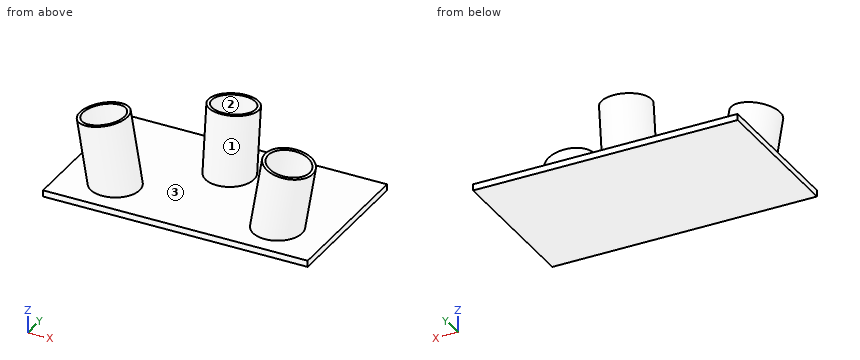
from build123d import *

# Parameters (mm, degrees)
F2_R      = 9.70750027
F2_R_2    = 8.43750027
F3_DEPTH  = 33.02
F4_DEPTH  = 50.8
F6_DEPTH  = 127
F8_R      = 9.70750027
F8_R_2    = 8.43750027
F9_DEPTH  = 33.02
F10_W     = 144.2738771439
F10_H     = 43.9907349646
F11_DEPTH = 381
F14_R     = 9.70750027
F14_R_2   = 8.43750027
F15_DEPTH = 25.4
F16_DEPTH = 50.8
F17_W     = 94.1894035786
F17_H     = 29.3832402676
F18_DEPTH = 127
F19_W     = 106.1688474409
F19_H     = 60.55200234
F20_DEPTH = 2.54


with BuildPart() as f3:
    # F2 (on line) → F3 (new body)
    with BuildSketch(Plane(origin=(0, 0, 0), x_dir=(0.9860251287, 0, 0.1665966554), z_dir=(0.1665966554, 0, -0.9860251287))):
        with Locations((-32.11030027, 38.1445123341)):
            Circle(F2_R)
        with Locations((-32.11030027, 38.1445123341)):
            Circle(F2_R_2, mode=Mode.SUBTRACT)
    extrude(amount=-F3_DEPTH)

    # F4 (add): a face of the model
    f4_faces = [f3.faces().sort_by_distance(p)[0] for p in [
        (-46.4636912241, -38.1445123341, 25.6375864152),
    ]]
    extrude(f4_faces, amount=-F4_DEPTH)

    # F5 (on Front) → F6 (cut, symmetric)
    with BuildSketch(Plane.XZ):
        Polygon((43.3516763151, 0), (0, 0), (-49.4034710573, 0), (-49.4034710573, -35.2993682027), (43.3516763151, -35.2993682027), align=None)
    extrude(amount=F6_DEPTH, both=True, mode=Mode.SUBTRACT)



with BuildPart() as f9:
    # F8 (on line) → F9 (new body)
    with BuildSketch(Plane(origin=(0, 0, 0), x_dir=(0.9860251287, 0, -0.1665966554), z_dir=(-0.1665966554, 0, -0.9860251287))):
        with Locations((32.11030027, 38.14450207)):
            Circle(F8_R)
        with Locations((32.11030027, 38.14450207)):
            Circle(F8_R_2, mode=Mode.SUBTRACT)
    extrude(amount=-F9_DEPTH)

    # F10 (on Front) → F11 (cut, symmetric)
    with BuildSketch(Plane.XZ):
        with Locations((2.6571601629, -21.9953674823)):
            Rectangle(F10_W, F10_H)
    extrude(amount=F11_DEPTH, both=True, mode=Mode.SUBTRACT)


with BuildPart() as f15:
    # F14 (on face) → F15 (new body)
    with BuildSketch(Plane(origin=(0, 0, 0), x_dir=(1, 0, 0), z_dir=(0, 0.1114689322, 0.9937679192))):
        with Locations((0, -12.55230027)):
            Circle(F14_R)
        with Locations((0, -12.55230027)):
            Circle(F14_R_2, mode=Mode.SUBTRACT)
    extrude(amount=F15_DEPTH)

    # F16 (add): a face of the model
    f16_faces = [f15.faces().sort_by_distance(p)[0] for p in [
        (-9.4329306992, -9.642762442, 26.6408966545),
    ]]
    extrude(f16_faces, amount=-F16_DEPTH)

    # F17 (on Right) → F18 (cut, symmetric)
    with BuildSketch(Plane.YZ):
        with Locations((-17.9154733196, -14.6916201338)):
            Rectangle(F17_W, F17_H)
    extrude(amount=F18_DEPTH, both=True, mode=Mode.SUBTRACT)


with BuildPart() as f3_1:
    add(f3.part)

    add(f9.part)  # F20 merges F9

    add(f15.part)  # F20 merges F15
    # F19 (on Top) → F20 (join)
    with BuildSketch(Plane.XY):
        with Locations((0, -23.92600117)):
            Rectangle(F19_W, F19_H)
    extrude(amount=-F20_DEPTH)


solid = f3_1.part
Input: part model. Units: mm. Frame: model coordinates. Face numbers are marked on the shaded views. Coordinates: 2 decimals unless noted, no trailing zeros. Loops run counter-clockwise (first coordinate to the right, second up) from the corner with the lowest first, then second, coordinate; pieces in that order, holes last. Notation, with made-up numbers: (66.25, -2.5) -> (77.25, -2.5) arc R21 cw to (77.25, 14.5) -> close; hole circle Ø11 at (-12.5, -25.5). An arc over 180 degrees is marked (long way). Write item = value, one per line. Start each with the question number.
Item 1: Cut plane A-A, the plane x = 11. Return loops of the section in (y, z).
Item 2: First-contact query: P1, Ø5, axis at x = 33, y = -40.5, coming from the +Z side; P2, Ø3, axis at y = -37, z = 22.5, coming from the -X side; P3, Ø2, axis at y = -34.5, z = 6.5, coming from the +X side. Flat tips, straight axial feed; report the tip coordinate or a pass-through.
Item 3: Mould query, pull axis Y, two halves, no side actions, for the marked faces 1, 2 and 3. Classes: pulls with the +Y half, pulls with the -Y half, needs draft (parallel to the pull), parting line crosses it, or undercut.
Item 4: Material intervals for line 1 (X direction, y = -44, z = 6); line 2 (Z direction, x = -44, y = -49); line 3 (X direction, y = -45, z = 2), sorted ascending.
Item 5: Cut plane C-C, the plane y = -35.5. Return loops of the section in (x, z).
Item 6: Cut plane B-B, the plane z = 7.5. Count the separate pieces of the cut face and the enclosed holes in it, plus the area to 3 significant figures.
Item 7: Cut plane D-D, the plane y = -51. Return loops of the section in (x, z).
Ans:
q1.outline = (-54.2, -2.54) -> (6.35, -2.54) -> (6.35, 0) -> (-54.2, 0) -> close
q2.P1 = 0
q2.P2 = -46.43
q2.P3 = 43.18
q3.face_1 = parting line crosses it
q3.face_2 = undercut
q3.face_3 = needs draft
q4.line_1 = -41.43 to -39.74, -27.42 to -25.73, 25.73 to 27.42, 39.74 to 41.43
q4.line_2 = -2.54 to 0
q4.line_3 = -39.87 to -37.89, -27.91 to -25.93, 25.93 to 27.91, 37.89 to 39.87
q5.outline = (-53.08, -2.54) -> (53.08, -2.54) -> (53.08, 0) -> (42.04, 0) -> (46.37, 25.65) -> (45.06, 25.87) -> (40.69, 0) -> (24.44, 0) -> (29.26, 28.54) -> (27.95, 28.77) -> (23.09, 0) -> (-23.09, 0) -> (-27.95, 28.77) -> (-29.26, 28.54) -> (-24.44, 0) -> (-40.69, 0) -> (-45.06, 25.87) -> (-46.37, 25.65) -> (-42.04, 0) -> (-53.08, 0) -> close
q6.separate_pieces = 3
q6.enclosed_holes = 3
q6.area = 220 mm²
q7.outline = (-53.08, -2.54) -> (53.08, -2.54) -> (53.08, 0) -> (-53.08, 0) -> close
